```python
from build123d import *

# Parameters (mm, degrees)
SKETCH1_W         = 223.7486
SKETCH1_H         = 128.4986
SKETCH1_W_2       = 222.25
SKETCH1_H_2       = 127
BASE_DEPTH        = 2.54
SKETCH1_3_W       = 223.7486
SKETCH1_3_H       = 128.4986
SKETCH1_3_W_2     = 222.25
SKETCH1_3_H_2     = 127
WALLS_DEPTH       = 30.1625
HANDLE_DEPTH      = 120.65
HANDLE_DEPTH_BACK = 120.65


with BuildPart() as part:
    # Sketch1 → Base (new body)
    with BuildSketch(Plane(origin=(0, 0, 0), x_dir=(1, 0, 0), z_dir=(0, 1, 0))):
        with Locations((0, 63.5)):
            Rectangle(SKETCH1_W, SKETCH1_H)
        with Locations((0, 63.5)):
            Rectangle(SKETCH1_W_2, SKETCH1_H_2, mode=Mode.SUBTRACT)
        with Locations((0, 63.5)):
            Rectangle(SKETCH1_W_2, SKETCH1_H_2)
    extrude(amount=BASE_DEPTH)

    # Sketch1_3 → Walls (add)
    with BuildSketch(Plane(origin=(0, 0, 0), x_dir=(1, 0, 0), z_dir=(0, 1, 0))):
        with Locations((0, 63.5)):
            Rectangle(SKETCH1_3_W, SKETCH1_3_H)
        with Locations((0, 63.5)):
            Rectangle(SKETCH1_3_W_2, SKETCH1_3_H_2, mode=Mode.SUBTRACT)
    extrude(amount=WALLS_DEPTH)

    # Sketch2 → Handle (add, two sides)
    with BuildSketch(Plane(origin=(0, 0, 0), x_dir=(0, 0, -1), z_dir=(1, 0, 0))) as handle_sk:
        Polygon((0, 22.475414602), (0, 31.1785), (-8.89, 31.1785), (-8.89, 15.6845), (-7.874, 15.6845), (-7.874, 30.1625), (-1.016, 30.1625), (-1.016, 22.475414602), align=None)
    extrude(amount=HANDLE_DEPTH)
    extrude(handle_sk.sketch, amount=-HANDLE_DEPTH_BACK)


solid = part.part
```
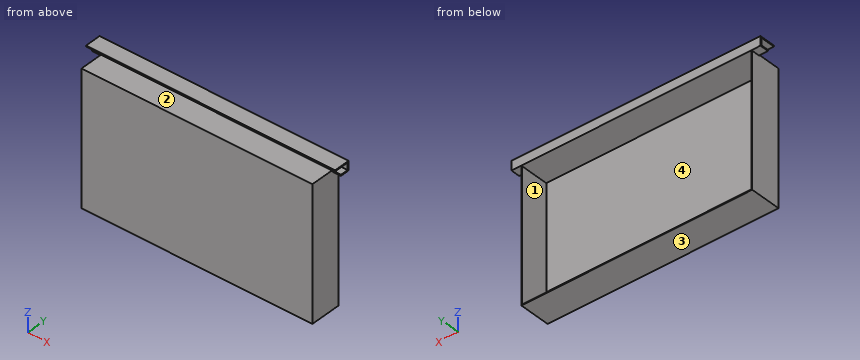
Can you work these out from the model? Positions are in its coordinate system, mm. Face numbers are marked on the shaded views. A direction names the side the tool comes from. Coordinates: 2 decimals unless noted, no trailing zeros. Loops run counter-clockwise (first coordinate to the right, second up) from the corner with the lowest first, then second, coordinate; pieces in that order, holes last.
1) For pin 1 (14 mm diameter, centred on y = 14.5, z = -84, fed in from -X); pin 2 (3 mm diameter, centred on y = 9, z = -22, fed in from +X); pin 3 (4 mm diameter, centred on x = -66.5, z = -18, fed in from +Y); pin 4 (12 mm diameter, centred on x = 36, y = 12.5, fed in from +Z), each with a flat end and sliding along its axis, tell me the tip position at first contact or that it passes through.
2) Which directions (+Z, -Z, +X, -X, +Y, -Y) give clear straight access to the entire face, cutting with the end or side of a thin tool? Please do the marked faces 3 and 4.
3) Imagine slicing it at D-D on x = -51. List the corners of the cut face in (y, z) for me, plus the area to 3 significant figures.
4) Imagine slicing it at A-A on y = 27. List the corners of the cut face in (x, z) for me (3 decimals).
5) Imagine slicing it at C-C on z = -87.5. List the corners of the cut face in (x, y) for me (1 decimal), plus the area to 3 significant figures.
6) I need wall thicknesses on probe 1 along Z at (x, y) = (35.5, 22); probe 2 along Z at (x, y) = (77, 25.5); probe 3 along X at (y, z) = (27, -36) (3 decimals). Which ranges of each line are inside material? Lowest first, please.
7) Thinking about a two-plate mould opening in X: for the marked faces 1 and 2, which applies, pulls with the +X half, pulls with the -X half, needs draft (parallel to the pull), parting line crosses it, or undercut?
8) Imagine slicing it at B-B on y = 9. List the corners of the cut face in (x, z) for me (3 decimals), plus the area to 3 significant figures.
Completed:
1. pin 1: stops at x = -111.87
1. pin 2: stops at x = 111.87
1. pin 3: stops at y = 2.54
1. pin 4: stops at z = 8.89
2. face 3: -Z, +X, -X, +Y, -Y
2. face 4: +Y
3. outline: (0, -127.75) - (30.16, -127.75) - (30.16, -127) - (2.54, -127) - (2.54, 0) - (31.18, 0) - (31.18, 8.89) - (15.68, 8.89) - (15.68, 7.87) - (30.16, 7.87) - (30.16, 1.02) - (22.48, 1.02) - (22.48, 0.75) - (0, 0.75) - close
3. area: 394 mm2
4. outline: (-120.65, 0) - (-111.874, 0) - (-111.874, -127.749) - (111.874, -127.749) - (111.874, 0) - (120.65, 0) - (120.65, 1.016) - (-120.65, 1.016) - close; (-120.65, 7.874) - (120.65, 7.874) - (120.65, 8.89) - (-120.65, 8.89) - close; hole (-111.125, -127) - (111.125, -127) - (111.125, 0) - (-111.125, 0) - close
5. outline: (-111.9, 0) - (111.9, 0) - (111.9, 30.2) - (111.1, 30.2) - (111.1, 2.5) - (-111.1, 2.5) - (-111.1, 30.2) - (-111.9, 30.2) - close
5. area: 610 mm2
6. probe 1: z = -127.75 to -127, 0 to 0.75, 7.87 to 8.89
6. probe 2: z = -127.75 to -127, 0 to 1.02, 7.87 to 8.89
6. probe 3: x = -111.874 to -111.125, 111.125 to 111.874
7. face 1: undercut
7. face 2: needs draft
8. outline: (-111.874, -127.749) - (111.874, -127.749) - (111.874, 0.749) - (-111.874, 0.749) - close; hole (-111.125, -127) - (111.125, -127) - (111.125, 0) - (-111.125, 0) - close
8. area: 526 mm2
